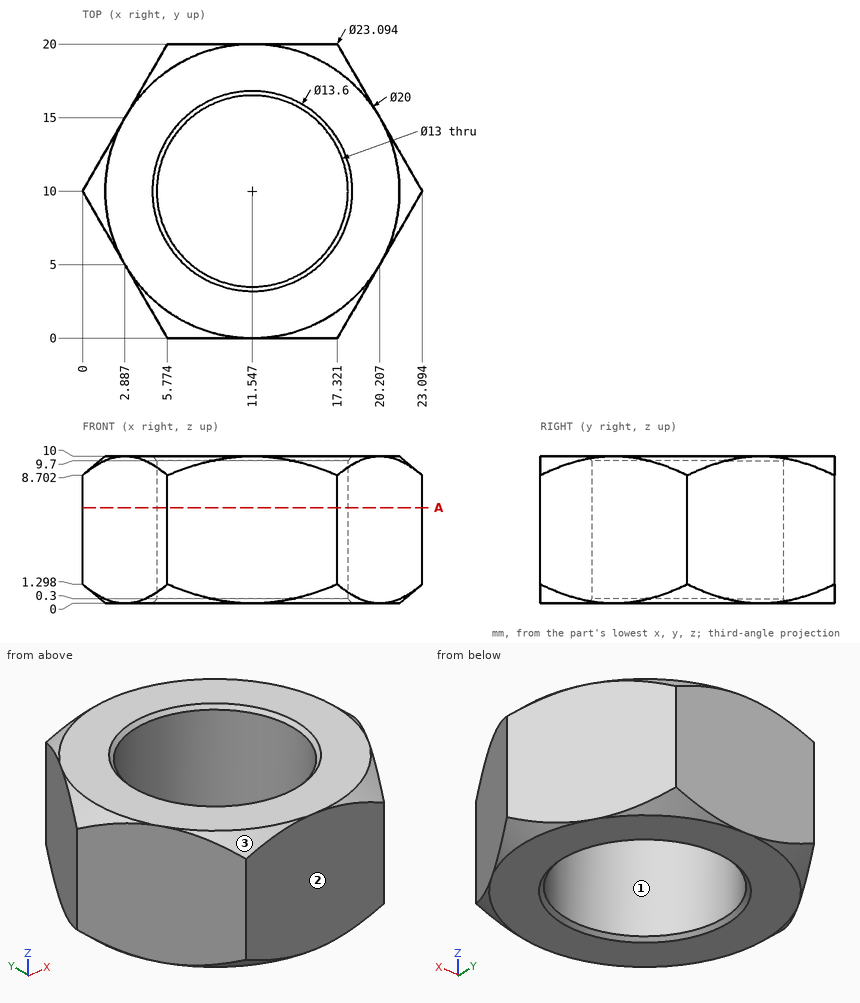
Could you check a few things on this drawing? It's one solid part, dimensions in mm from its lowest x, y, z. Coordinates: 2 decimals unless noted, no trailing zeros. Write each loop counter-clockwise with the first axis right and the second up, starting at its lowest first coordinate (ties: lowest second). Pieces come first, ordered by that corner, then holes.
1) If we section it at A-A (z = 6.5): List the corners of the cut face in (x, y) for me (1 decimal), plus the area to 3 significant figures.
Filled in:
outline: (0, 10) - (5.8, 0) - (17.3, 0) - (23.1, 10) - (17.3, 20) - (5.8, 20) - close; hole circle Ø13 at (11.5, 10)
area: 214 mm2
2) I'm going to push flat-ended pins straight in: pin 1 (10 mm diameter, centred on x = 9, y = 4.5, fed in from +Z); pin 2 (3 mm diameter, centred on y = 2, z = 1.5, fed in from +X); pin 3 (8 mm diameter, centred on x = 11.55, y = 10, fed in from +Z). Where does each tip first touch, or does it pass through?
Filled in:
pin 1: stops at z = 10
pin 2: stops at x = 19.34
pin 3: passes through
3) If I drill on line 1 (Y direction, x = 11.75, z = 4); line 2 (Y direction, x = 17, z = 7.5) (1 decimal); line 3 (X direction, y = 18.5, z = 0.5) (1 decimal), over which ranges is the centre line in solid material (lowest first)?
Filled in:
line 1: y = 0 to 3.5, 16.5 to 20
line 2: y = 0 to 6.5, 13.5 to 20
line 3: x = 5.2 to 17.9
4) Thinking about a two-plate mould opening in X: for the marked faces 1, 2 and 3, which applies, +X half, -X half, draft (parallel to the pull), parting line (faces both ways), or undercut?
Filled in:
face 1: undercut
face 2: draft
face 3: -X half
